The model under review builds one solid part; all positions refer to its coordinate system, in mm. Coordinates: 2 decimals unless noted, no trailing zeros. Use CSV: the item, a comma, the result in double quotes. Start each with the question number.
1. Draft analysis for pull direction X (two halves, no side actions). For faces 1 (the flat face through (-8.077, -2.324, 1.014)), 2 (the flat face through (3, 0, 2)), state which applies: +X half, -X half, draft (parallel to the pull), parting line (faces both ways), or undercut.
2. For L1, parallel to X at y = -8.5, z = 1.25; L2, parallel to X at y = 3, z = 0.5; L3, parallel to Y at x = -6.5, z = 0.7, list the stretches that pass through material, from the lowest coordinate up.
3. Add section A-A, the plane x = 0. State how many separate pieces and enclosed holes the cut face has, then the cut area to 3 significant figures.
from build123d import *

# Parameters (mm, degrees)
SKETCH1_R           = 12.5
BOSS_EXTRUDE1_DEPTH = 2
CUT_EXTRUDE1_DEPTH  = 2
CUT_EXTRUDE2_DEPTH  = 2


with BuildPart() as part:
    # Sketch1 → Boss-Extrude1 (new body)
    with BuildSketch(Plane.XY):
        Circle(SKETCH1_R)
    extrude(amount=BOSS_EXTRUDE1_DEPTH)

    # Sketch2 → Cut-Extrude1 (cut)
    with BuildSketch(Plane.XY.offset(2)):
        with BuildLine():
            Line((1.85, 2.101784956), (1.85, -2.101784956))
            ThreePointArc((1.85, -2.101784956), (0, -2.8), (-1.85, -2.101784956))
            Line((-1.85, -2.101784956), (-1.85, 2.101784956))
            ThreePointArc((-1.85, 2.101784956), (0, 2.8), (1.85, 2.101784956))
        make_face()
    extrude(amount=-CUT_EXTRUDE1_DEPTH, mode=Mode.SUBTRACT)

    # Sketch3 → Cut-Extrude2 (cut)
    with BuildSketch(Plane.XY.offset(2)):
        with BuildLine():
            Line((-0.575541349, 5.8), (0.575541349, 5.8))
            Line((0.575541349, 5.8), (1.323383427, 10.975313802))
            add(Edge.make_bspline(
                [(-1.323383427, 10.975313802), (0, 11.388369724), (1.323383427, 10.975313802)],
                knots=[0, 0, 0, 1, 1, 1], degree=2))
            Line((-1.323383427, 10.975313802), (-0.575541349, 5.8))
        make_face()
        with BuildLine():
            Line((2.75129478, 5.13825115), (5.422717619, 9.633430872))
            add(Edge.make_bspline(
                [(2.977423895, 10.646304697), (4.358140415, 10.521481696), (5.422717619, 9.633430872)],
                knots=[0, 0, 0, 1, 1, 1], degree=2))
            Line((2.977423895, 10.646304697), (1.687833035, 5.578751427))
            Line((1.687833035, 5.578751427), (2.75129478, 5.13825115))
        make_face()
        with BuildLine():
            Line((4.508188522, 3.69425014), (8.69649221, 6.82494542))
            add(Edge.make_bspline(
                [(6.82494542, 8.69649221), (8.052793458, 8.052793458), (8.69649221, 6.82494542)],
                knots=[0, 0, 0, 1, 1, 1], degree=2))
            Line((6.82494542, 8.69649221), (3.69425014, 4.508188522))
            Line((3.69425014, 4.508188522), (4.508188522, 3.69425014))
        make_face()
        with BuildLine():
            Line((5.578751427, 1.687833035), (10.646304697, 2.977423895))
            add(Edge.make_bspline(
                [(9.633430872, 5.422717619), (10.521481696, 4.358140415), (10.646304697, 2.977423895)],
                knots=[0, 0, 0, 1, 1, 1], degree=2))
            Line((9.633430872, 5.422717619), (5.13825115, 2.75129478))
            Line((5.13825115, 2.75129478), (5.578751427, 1.687833035))
        make_face()
        with BuildLine():
            Line((5.8, -0.575541349), (10.975313802, -1.323383427))
            add(Edge.make_bspline(
                [(10.975313802, 1.323383427), (11.388369724, 0), (10.975313802, -1.323383427)],
                knots=[0, 0, 0, 1, 1, 1], degree=2))
            Line((10.975313802, 1.323383427), (5.8, 0.575541349))
            Line((5.8, 0.575541349), (5.8, -0.575541349))
        make_face()
        with BuildLine():
            Line((5.13825115, -2.75129478), (9.633430872, -5.422717619))
            add(Edge.make_bspline(
                [(10.646304697, -2.977423895), (10.521481696, -4.358140415), (9.633430872, -5.422717619)],
                knots=[0, 0, 0, 1, 1, 1], degree=2))
            Line((10.646304697, -2.977423895), (5.578751427, -1.687833035))
            Line((5.578751427, -1.687833035), (5.13825115, -2.75129478))
        make_face()
        with BuildLine():
            Line((3.69425014, -4.508188522), (6.82494542, -8.69649221))
            add(Edge.make_bspline(
                [(8.69649221, -6.82494542), (8.052793458, -8.052793458), (6.82494542, -8.69649221)],
                knots=[0, 0, 0, 1, 1, 1], degree=2))
            Line((8.69649221, -6.82494542), (4.508188522, -3.69425014))
            Line((4.508188522, -3.69425014), (3.69425014, -4.508188522))
        make_face()
        with BuildLine():
            Line((1.687833035, -5.578751427), (2.977423895, -10.646304697))
            add(Edge.make_bspline(
                [(5.422717619, -9.633430872), (4.358140415, -10.521481696), (2.977423895, -10.646304697)],
                knots=[0, 0, 0, 1, 1, 1], degree=2))
            Line((5.422717619, -9.633430872), (2.75129478, -5.13825115))
            Line((2.75129478, -5.13825115), (1.687833035, -5.578751427))
        make_face()
        with BuildLine():
            Line((-0.575541349, -5.8), (-1.323383427, -10.975313802))
            add(Edge.make_bspline(
                [(1.323383427, -10.975313802), (0, -11.388369724), (-1.323383427, -10.975313802)],
                knots=[0, 0, 0, 1, 1, 1], degree=2))
            Line((1.323383427, -10.975313802), (0.575541349, -5.8))
            Line((0.575541349, -5.8), (-0.575541349, -5.8))
        make_face()
        with BuildLine():
            Line((-2.75129478, -5.13825115), (-5.422717619, -9.633430872))
            add(Edge.make_bspline(
                [(-2.977423895, -10.646304697), (-4.358140415, -10.521481696), (-5.422717619, -9.633430872)],
                knots=[0, 0, 0, 1, 1, 1], degree=2))
            Line((-2.977423895, -10.646304697), (-1.687833035, -5.578751427))
            Line((-1.687833035, -5.578751427), (-2.75129478, -5.13825115))
        make_face()
        with BuildLine():
            Line((-4.508188522, -3.69425014), (-8.69649221, -6.82494542))
            add(Edge.make_bspline(
                [(-6.82494542, -8.69649221), (-8.052793458, -8.052793458), (-8.69649221, -6.82494542)],
                knots=[0, 0, 0, 1, 1, 1], degree=2))
            Line((-6.82494542, -8.69649221), (-3.69425014, -4.508188522))
            Line((-3.69425014, -4.508188522), (-4.508188522, -3.69425014))
        make_face()
        with BuildLine():
            Line((-5.578751427, -1.687833035), (-10.646304697, -2.977423895))
            add(Edge.make_bspline(
                [(-9.633430872, -5.422717619), (-10.521481696, -4.358140415), (-10.646304697, -2.977423895)],
                knots=[0, 0, 0, 1, 1, 1], degree=2))
            Line((-9.633430872, -5.422717619), (-5.13825115, -2.75129478))
            Line((-5.13825115, -2.75129478), (-5.578751427, -1.687833035))
        make_face()
        with BuildLine():
            Line((-5.8, 0.575541349), (-10.975313802, 1.323383427))
            add(Edge.make_bspline(
                [(-10.975313802, -1.323383427), (-11.388369724, 0), (-10.975313802, 1.323383427)],
                knots=[0, 0, 0, 1, 1, 1], degree=2))
            Line((-10.975313802, -1.323383427), (-5.8, -0.575541349))
            Line((-5.8, -0.575541349), (-5.8, 0.575541349))
        make_face()
        with BuildLine():
            Line((-5.13825115, 2.75129478), (-9.633430872, 5.422717619))
            add(Edge.make_bspline(
                [(-10.646304697, 2.977423895), (-10.521481696, 4.358140415), (-9.633430872, 5.422717619)],
                knots=[0, 0, 0, 1, 1, 1], degree=2))
            Line((-10.646304697, 2.977423895), (-5.578751427, 1.687833035))
            Line((-5.578751427, 1.687833035), (-5.13825115, 2.75129478))
        make_face()
        with BuildLine():
            Line((-3.69425014, 4.508188522), (-6.82494542, 8.69649221))
            add(Edge.make_bspline(
                [(-8.69649221, 6.82494542), (-8.052793458, 8.052793458), (-6.82494542, 8.69649221)],
                knots=[0, 0, 0, 1, 1, 1], degree=2))
            Line((-8.69649221, 6.82494542), (-4.508188522, 3.69425014))
            Line((-4.508188522, 3.69425014), (-3.69425014, 4.508188522))
        make_face()
        with BuildLine():
            Line((-1.687833035, 5.578751427), (-2.977423895, 10.646304697))
            add(Edge.make_bspline(
                [(-5.422717619, 9.633430872), (-4.358140415, 10.521481696), (-2.977423895, 10.646304697)],
                knots=[0, 0, 0, 1, 1, 1], degree=2))
            Line((-5.422717619, 9.633430872), (-2.75129478, 5.13825115))
            Line((-2.75129478, 5.13825115), (-1.687833035, 5.578751427))
        make_face()
    extrude(amount=-CUT_EXTRUDE2_DEPTH, mode=Mode.SUBTRACT)


solid = part.part
Computed:
1,face 1,"undercut"
1,face 2,"draft"
2,L1,"x = -9.17 to -7.16, -6.68 to -4.75, -2.43 to -0.97, 0.97 to 2.43, 4.75 to 6.68, 7.16 to 9.17"
2,L2,"x = -12.13 to -10.64, -5.56 to 5.56, 10.64 to 12.13"
2,L3,"y = -10.68 to -8.26, -5.18 to -3.56, -1.92 to -0.68, 0.68 to 1.92, 3.56 to 5.18, 8.26 to 10.68"
3,separate pieces,"4"
3,enclosed holes,"0"
3,area,"17.3 mm^2"
